```python
from build123d import *

# Parameters (mm, degrees)
SKETCH_1_W      = 15
SKETCH_1_H      = 120
SKETCH_1_R      = 1.5
SKETCH_1_R_2    = 4
EXTRUDE_1_DEPTH = 1.75
FILLET_1_R      = 3
FILLET_2_R      = 6


with BuildPart() as part:
    # 草图1 → 凸台-拉伸1 (new body)
    # profile 1 of 3: a face of its own
    with BuildSketch(Plane.XY):
        with BuildLine():
            ThreePointArc((56.291651246, 32.5), (0, 65), (-56.291651246, 32.5))
            Line((-56.291651246, 32.5), (-69.282032303, 40))
            ThreePointArc((-69.282032303, 40), (0, 80), (69.282032303, 40))
            Line((69.282032303, 40), (56.291651246, 32.5))
        make_face()
    # profile 2 of 3: a face of its own
    with BuildSketch(Plane.XY):
        with Locations((0, 4.565857851)):
            Rectangle(SKETCH_1_W, SKETCH_1_H)
        with Locations((0, 49.565857851)):
            Circle(SKETCH_1_R, mode=Mode.SUBTRACT)
        with Locations((0, 29.565857851)):
            Circle(SKETCH_1_R, mode=Mode.SUBTRACT)
        with Locations((0, 39.565857851)):
            Circle(SKETCH_1_R_2, mode=Mode.SUBTRACT)
        with Locations((0, -26.434142149)):
            Circle(SKETCH_1_R, mode=Mode.SUBTRACT)
        with Locations((5, -43.434142149)):
            Circle(SKETCH_1_R, mode=Mode.SUBTRACT)
        with Locations((-5, -43.434142149)):
            Circle(SKETCH_1_R, mode=Mode.SUBTRACT)
        with Locations((0, -50.434142149)):
            Circle(SKETCH_1_R, mode=Mode.SUBTRACT)
    # profile 3 of 3: a face of its own
    with BuildSketch(Plane.XY):
        with BuildLine():
            ThreePointArc((7.5, 64.565857851), (0, 65), (-7.5, 64.565857851))
            Line((-7.5, 64.565857851), (7.5, 64.565857851))
        make_face()
    extrude(amount=EXTRUDE_1_DEPTH)

    # 圆角1
    fillet_1_edges = [part.edges().sort_by_distance(p)[0] for p in [
        (7.5, -55.434142149, 0.875),
        (-7.5, -55.434142149, 0.875),
        (-56.291651246, 32.5, 0.875),
        (-69.282032303, 40, 0.875),
        (69.282032303, 40, 0.875),
        (56.291651246, 32.5, 0.875),
    ]]
    fillet(fillet_1_edges, radius=FILLET_1_R)

    # 圆角2
    fillet_2_edges = [part.edges().sort_by_distance(p)[0] for p in [
        (7.5, 64.565857851, 0.875),
        (-7.5, 64.565857851, 0.875),
    ]]
    fillet(fillet_2_edges, radius=FILLET_2_R)


solid = part.part
```
The listing builds one solid part. Answer for the finished solid, in the listing's coordinates (mm). A direction names the side the tool comes from. Coordinates: 2 decimals unless noted, no trailing zeros. Write each loop counter-clockwise with the first axis right and the second up, starting at its lowest first coordinate (ties: lowest second). Pieces come first, ordered by that corner, then holes. Notation, with made-up numbers: M 0.25,76.25 L 19.25,76.25 A17 cw 19.25,102.25 Z; hole C 75.25,54 d2. An arc over 180 degrees is marked long. Use a Markdown table: item, result. Add a question column.
1. Which of the six approach directions +Z, -Z, +X, -X, +Y, -Y give full straight-line access (tool end or side, diameter ignored) to faces 4 (the cylindrical face through (-0.325, -51.898, 0.863)), 5 (the cylindrical face through (37.892, 52.813, 0.863))?
2. Section A-A (z = 1.2) is taken. Give the vertices of the cut face in (x, y), plus the area to 3 significant figures.
3. Straight lines are drawn through the part: line 1 along Y through (x, z) = (0, 0.65); line 2 along Y through (x, z) = (0.5, 1.2); line 3 along X through (y, z) = (59.5, 0.75). For each, find the intervals that lie inside material, in ascending order. Write a range as [from, to].
4. For a pull along X with two mould halves and no side action, classify faces 1 (the cylindrical face through (-0.195, 31.053, 0.863)), 2 (the flat face through (0, 33, 1.75)), 3 (the flat face through (62.79, 36.25, 0.86)) as +X half, -X half, draft (parallel to the pull), parting line (faces both ways), or undercut.
5. Section B-B (y = -36.5) is taken. Give the vertices of the cut face in (x, z).
6. Section C-C (x = 19) is taken. Give the vertices of the cut face in (y, z).
7. Given P1, Ø5, axis at x = 0, y = -26.43, coming from the -Z side; P2, Ø2.5, axis at x = -5, y = -43.43, coming from the +Z side; P3, Ø0.5, axis at y = 1, z = 1, coming from the +X side, each flat-ended and moving along its own axis, determine where each tip first touches the part or whether it passes through.
Data:
| question | item | result |
|---|---|---|
| 1 | face 4 | +Z, -Z |
| 1 | face 5 | +Z, -Z, -Y |
| 2 | outline | M -67.67,42.67 A3 ccw -66.63,38.47 L -58.83,33.97 A3 ccw -54.8,34.95 A65 cw -14.87,63.28 A6 cw -7.5,57.43 L -7.5,-52.43 A3 ccw -4.5,-55.43 L 4.5,-55.43 A3 ccw 7.5,-52.43 L 7.5,57.43 A6 cw 14.87,63.28 A65 cw 54.8,34.95 A3 ccw 58.83,33.97 L 66.63,38.47 A3 ccw 67.67,42.67 A80 ccw Z; hole C -5,-43.43 d3; hole C 0,39.57 d8; hole C 0,-50.43 d3; hole C 0,-26.43 d3; hole C 0,29.57 d3; hole C 0,49.57 d3; hole C 5,-43.43 d3 |
| 2 | area | 4,000 mm2 |
| 3 | line 1 | y = [-55.43, -51.93], [-48.93, -27.93], [-24.93, 28.07], [31.07, 35.57], [43.57, 48.07], [51.07, 80] |
| 3 | line 2 | y = [-55.43, -51.85], [-49.02, -27.85], [-25.02, 28.15], [30.98, 35.6], [43.53, 48.15], [50.98, 80] |
| 3 | line 3 | x = [-53.48, -26.17], [-7.87, 7.87], [26.17, 53.48] |
| 4 | face 1 | undercut |
| 4 | face 2 | draft |
| 4 | face 3 | +X half |
| 5 | outline | M -7.5,0 L 7.5,0 L 7.5,1.75 L -7.5,1.75 Z |
| 6 | outline | M 62.16,0 L 77.71,0 L 77.71,1.75 L 62.16,1.75 Z |
| 7 | P1 | stops at z = 0 |
| 7 | P2 | passes through |
| 7 | P3 | stops at x = 7.5 |
